Build history of the part. All positions in model axes, mm. A direction names the side the tool comes from. Give positions to 0.01 mm unless a question says otherwise; leave off trailing zeros. Write each loop counter-clockwise with the first axis right and the second up, starting at its lowest first coordinate (ties: lowest second). Pieces come first, ordered by that corner, then holes.
from build123d import *

# Parameters (mm, degrees)
SKETCH1_R           = 2
SKETCH1_R_2         = 2.5
SKETCH1_W           = 4
SKETCH1_H           = 7.5
SKETCH1_H_2         = 6
SKETCH1_W_2         = 10
SKETCH1_H_3         = 4
BOSS_EXTRUDE1_DEPTH = 4


with BuildPart() as part:
    # Sketch1 → Boss-Extrude1 (new body)
    with BuildSketch(Plane(origin=(0, 0, 0), x_dir=(1, 0, 0), z_dir=(0, 1, 0))):
        Polygon((80, 124.45742592), (-80, 124.45742592), (-100, 104.45742592), (-100, 29.45742592), (-80, 9.45742592), (-80, -10.54257408), (-100, -30.54257408), (-100, -105.54257408), (-80, -125.54257408), (80, -125.54257408), (100, -105.54257408), (100, -30.54257408), (80, -10.54257408), (80, 9.45742592), (100, 29.45742592), (100, 104.45742592), align=None)
        with Locations(Location((-85, 94.45742592, 0), (0, 0, 270))):
            Circle(SKETCH1_R, mode=Mode.SUBTRACT)
        with Locations(Location((-85, 46.45742592, 0), (0, 0, 270))):
            Circle(SKETCH1_R, mode=Mode.SUBTRACT)
        with Locations(Location((85, 94.45742592, 0), (0, 0, 90))):
            Circle(SKETCH1_R, mode=Mode.SUBTRACT)
        with Locations(Location((85, 46.45742592, 0), (0, 0, 90))):
            Circle(SKETCH1_R, mode=Mode.SUBTRACT)
        with Locations(Location((85, -47.54257408, 0), (0, 0, 270))):
            Circle(SKETCH1_R, mode=Mode.SUBTRACT)
        with Locations(Location((85, -95.54257408, 0), (0, 0, 270))):
            Circle(SKETCH1_R, mode=Mode.SUBTRACT)
        with Locations(Location((-85, -47.54257408, 0), (0, 0, 90))):
            Circle(SKETCH1_R, mode=Mode.SUBTRACT)
        with Locations(Location((-85, -95.54257408, 0), (0, 0, 90))):
            Circle(SKETCH1_R, mode=Mode.SUBTRACT)
        with Locations(Location((60, 114.45742592, 0), (0, 0, 270))):
            Circle(SKETCH1_R_2, mode=Mode.SUBTRACT)
        with Locations(Location((-60, 114.45742592, 0), (0, 0, 90))):
            Circle(SKETCH1_R_2, mode=Mode.SUBTRACT)
        with Locations(Location((-75, -115.54257408, 0), (0, 0, 270))):
            Circle(SKETCH1_R, mode=Mode.SUBTRACT)
        with Locations(Location((-70, -10.54257408, 0), (0, 0, 270))):
            Circle(SKETCH1_R, mode=Mode.SUBTRACT)
        with Locations(Location((75, -115, 0), (0, 0, 270))):
            Circle(SKETCH1_R, mode=Mode.SUBTRACT)
        with Locations(Location((70, -10.54257408, 0), (0, 0, 270))):
            Circle(SKETCH1_R, mode=Mode.SUBTRACT)
        with BuildLine():
            Line((-20, 29.45742592), (20, 29.45742592))
            ThreePointArc((20, 29.45742592), (27.071067812, 26.528493731), (30, 19.45742592))
            Line((30, 19.45742592), (30, -40.54257408))
            ThreePointArc((30, -40.54257408), (27.071067812, -47.613641892), (20, -50.54257408))
            Line((20, -50.54257408), (-20, -50.54257408))
            ThreePointArc((-20, -50.54257408), (-27.071067812, -47.613641892), (-30, -40.54257408))
            Line((-30, -40.54257408), (-30, 19.45742592))
            ThreePointArc((-30, 19.45742592), (-27.071067812, 26.528493731), (-20, 29.45742592))
        make_face(mode=Mode.SUBTRACT)
        with BuildLine():
            Line((20, -73.04257408), (-20, -73.04257408))
            ThreePointArc((-20, -73.04257408), (-22.5, -75.54257408), (-20, -78.04257408))
            Line((-20, -78.04257408), (20, -78.04257408))
            ThreePointArc((20, -78.04257408), (22.5, -75.54257408), (20, -73.04257408))
        make_face(mode=Mode.SUBTRACT)
        with Locations((95, -41.25)):
            Rectangle(SKETCH1_W, SKETCH1_H, mode=Mode.SUBTRACT)
        with Locations((95, -96.822248533)):
            Rectangle(SKETCH1_W, SKETCH1_H_2, mode=Mode.SUBTRACT)
        with Locations((70, 8)):
            Rectangle(SKETCH1_W_2, SKETCH1_H_3, mode=Mode.SUBTRACT)
        with Locations((95, -56.25)):
            Rectangle(SKETCH1_W, SKETCH1_H, mode=Mode.SUBTRACT)
        with Locations((50, 8)):
            Rectangle(SKETCH1_W_2, SKETCH1_H_3, mode=Mode.SUBTRACT)
        with Locations((95, -84.822248533)):
            Rectangle(SKETCH1_W, SKETCH1_H_2, mode=Mode.SUBTRACT)
        with Locations((-95, -96.822248533)):
            Rectangle(SKETCH1_W, SKETCH1_H_2, mode=Mode.SUBTRACT)
        with Locations((-95, -84.822248533)):
            Rectangle(SKETCH1_W, SKETCH1_H_2, mode=Mode.SUBTRACT)
        with Locations((-95, -56.25)):
            Rectangle(SKETCH1_W, SKETCH1_H, mode=Mode.SUBTRACT)
        with Locations((-95, -41.25)):
            Rectangle(SKETCH1_W, SKETCH1_H, mode=Mode.SUBTRACT)
        with Locations((-50, 8)):
            Rectangle(SKETCH1_W_2, SKETCH1_H_3, mode=Mode.SUBTRACT)
        with Locations((-70, 8)):
            Rectangle(SKETCH1_W_2, SKETCH1_H_3, mode=Mode.SUBTRACT)
        with BuildLine():
            Line((20, 51.95742592), (-20, 51.95742592))
            ThreePointArc((-20, 51.95742592), (-22.5, 54.45742592), (-20, 56.95742592))
            Line((-20, 56.95742592), (20, 56.95742592))
            ThreePointArc((20, 56.95742592), (22.5, 54.45742592), (20, 51.95742592))
        make_face(mode=Mode.SUBTRACT)
    extrude(amount=BOSS_EXTRUDE1_DEPTH)


solid = part.part
(1) Drop flat-ended pins along their axis: pin 1 (4 mm diameter, centred on x = 8.5, z = 68.5, fed in from -Y); pin 2 (1.2 mm diameter, centred on y = 2, z = 0, fed in from -X); pin 3 (2 mm diameter, centred on x = 95.5, y = 2, fed in from -Z); pin 4 (2 mm diameter, centred on y = 2, z = 17, fed in from -X). Give the stop position or say it passes through.
(2) Saw through at A-A, the plane x = 5. List the corners of the cut face in (y, z).
(3) 3-axis set-ups, long thin cutter, end or side, ignore diameter. For faces 5 (the face through (-90.14, 1.97, -19.6)), 6 (the face through (27, 2, -26.6)), 7 (the face through (-24, 0, -29)): which of +Z, -Z, +X, -X, +Y, -Y reach the whole face in a straight line?
(4) Mould opens along Z. For faces 1 (the face through (89.86, 1.97, -19.32)), 2 (the face through (-89.86, 1.97, -114.6)), 3 (the face through (-24, 4, -29)), 4 (the face through (90.14, 1.97, 20.68)) say: +Z half, -Z half, draft (parallel to the pull), parting line (faces both ways), or undercut.
(5) Probe line 1 (X direction, y = 2.1, z = -9.5); line 2 (Z direction, x = 69.5, y = 2.1); line 3 (X direction, y = 3, z = 59.5). List the from-to ranges inside material, lowest first.
(6) Saw through at B-B, the plane y = 1.4. Give the number of separate pieces and of enclosed holes in the cut face, plus the area to 3 significant figures.
Computed values:
1. pin 1: stops at y = 0
1. pin 2: stops at x = -80
1. pin 3: stops at z = -109.96
1. pin 4: stops at x = -87.46
2. outline: (0, -124.46) - (4, -124.46) - (4, -56.96) - (0, -56.96) - close; (0, -51.96) - (4, -51.96) - (4, -29.46) - (0, -29.46) - close; (0, 50.54) - (4, 50.54) - (4, 73.04) - (0, 73.04) - close; (0, 78.04) - (4, 78.04) - (4, 125.54) - (0, 125.54) - close
3. face 5: -X, +Y, -Y
3. face 6: +Y, -Y
3. face 7: +Z, -Z, +X, -X, -Y
4. face 1: undercut
4. face 2: -Z half
4. face 3: draft
4. face 4: undercut
5. line 1: x = -80.04 to -75, -65 to -55, -45 to -30, 30 to 45, 55 to 65, 75 to 80.04
5. line 2: z = -124.46 to -10, -6 to 8.61, 12.48 to 125.54
5. line 3: x = -100 to -97, -93 to 93, 97 to 100
6. separate pieces: 1
6. enclosed holes: 29
6. area: 41,900 mm2
